from build123d import *

# Parameters (mm, degrees)
BOSS_EXTRUDE1_DEPTH = 4
BOSS_EXTRUDE2_DEPTH = 4
SKETCH3_R           = 1.25
BOSS_EXTRUDE3_DEPTH = 15
FILLET1_R           = 1
FILLET2_R           = 0.5
FILLET3_R           = 0.75


with BuildPart() as part:
    # Sketch1 → Boss-Extrude1 (new body)
    with BuildSketch(Plane.XY):
        Polygon((2.3, -4.75), (3.5, -4.75), (3.5, 4.75), (2.3, 4.75), (2.3, 2.65), (-0.2, 2.65), (-0.2, 4.75), (-3.5, 4.75), (-3.5, -4.75), (-0.2, -4.75), (-0.2, -2.65), (2.3, -2.65), align=None)
    extrude(amount=BOSS_EXTRUDE1_DEPTH)

    # Sketch2 → Boss-Extrude2 (add)
    with BuildSketch(Plane(origin=(0, 0, 0), x_dir=(-1, 0, 0), z_dir=(0, 0, -1))):
        Polygon((-7.5, 2.5), (-7.5, -2.5), (-3.5, -4.75), (-3.5, 4.75), align=None)
    extrude(amount=-BOSS_EXTRUDE2_DEPTH)

    # Sketch3 → Boss-Extrude3 (add)
    with BuildSketch(Plane.XY.offset(4)):
        with Locations((-1.5, 0)):
            Circle(SKETCH3_R)
    extrude(amount=BOSS_EXTRUDE3_DEPTH)

    # Fillet1
    fillet1_edges = [part.edges().sort_by_distance(p)[0] for p in [
        (-3.5, -4.75, 2),
        (-3.5, 4.75, 2),
        (3.5, 4.75, 2),
        (3.5, -4.75, 2),
        (7.5, -2.5, 2),
        (7.5, 2.5, 2),
    ]]
    fillet(fillet1_edges, radius=FILLET1_R)

    # Fillet2
    fillet2_edges = [part.edges().sort_by_distance(p)[0] for p in [
        (-2.75, 0, 4),
    ]]
    fillet(fillet2_edges, radius=FILLET2_R)

    # Fillet3
    fillet3_edges = [part.edges().sort_by_distance(p)[0] for p in [
        (-2.75, 0, 19),
    ]]
    fillet(fillet3_edges, radius=FILLET3_R)


solid = part.part
Geometry check sheet. Reference: the model listing, model coordinates, mm. A direction names the side the tool comes from. Round coordinates to 2 decimals unless told otherwise and drop trailing zeros. Loops run counter-clockwise (first coordinate to the right, second up) from the corner with the lowest first, then second, coordinate; pieces in that order, holes last. Notation, with made-up numbers: (18.25, 38.5) -> (77.25, 38.5) arc R22 ccw to (77.25, 47.5) -> close; hole circle Ø8 at (-32.75, 18.25). An arc over 180 degrees is marked (long way). Answer as a JSON object with one key per item and string values. Group by question number.
Item 1: Cross-section at C-C, the plane z = 14.5. Record the cut outline in (x, y).
Item 2: Cross-section at A-A, the plane z = 2.5. Record the cut outline in (x, y).
Item 3: Thickness scan on line 1 along Z through (x, y) = (4.5, 3.25); line 2 along Y through (x, z) = (-1.5, 6.25); line 3 along X through (y, z) = (-0.75, 13). Record the ranges inside material, lowest first.
Item 4: Cross-section at D-D, the plane x = 2.75. Record the cut outline in (y, z), plus the area to 3 significant figures.
Item 5: Set-up check for faces 1 (the face through (1, 2.65, 2)), 2 (the face through (3, 4.75, 2)), 3 (the face through (5.382, -3.691, 1.972)), 4 (the face through (-0.31, 0.38, 11.28)), 5 (the face through (-0.2, -4, 2)): record each of +Z, -Z, +X, -X, +Y, -Y from which the full face is reachable in a straight line by a thin tool's end or side.
Item 6: Cross-section at B-B, the plane x = 1.5. Record the cut outline in (y, z), plus the area to 3 significant figures.
Item 7: Release check for a two-part mould opening along X. For faces 6 (the face through (2, 0, 0)), 7 (the face through (2.3, -4, 2)), 8 (the face through (7.5, 0, 2)), 9 (the face through (-0.2, 4, 2)) record: pulls with the +X half, pulls with the -X half, needs draft (parallel to the pull), parting line crosses it, or undercut.
Item 8: Depth check by flat-ended pin: pin 1 Ø4 at (y, z) = (-1, 8.5) entering from +X; pin 2 Ø5 at (x, y) = (-0.5, 2) entering from +Z; pin 3 Ø2 at (x, z) = (1, 3) entering from +Y; pin 4 Ø1 at (x, y) = (-2, -1.5) entering from +Z. Enter the tip coordinate at first touch or a pass-through.
Determined:
{
 "1": {"outline": "circle Ø2.5 at (-1.5, 0)"},
 "2": {"outline": "(-3.5, -3.75) arc R1 ccw to (-2.5, -4.75) -> (-0.2, -4.75) -> (-0.2, -2.65) -> (2.3, -2.65) -> (2.3, -4.75) -> (3.24, -4.75) arc R1 ccw to (3.73, -4.62) -> (6.99, -2.79) arc R1 ccw to (7.5, -1.92) -> (7.5, 1.92) arc R1 ccw to (6.99, 2.79) -> (3.73, 4.62) arc R1 ccw to (3.24, 4.75) -> (2.3, 4.75) -> (2.3, 2.65) -> (-0.2, 2.65) -> (-0.2, 4.75) -> (-2.5, 4.75) arc R1 ccw to (-3.5, 3.75) -> close"},
 "3": {"line 1": "z = 0 to 4", "line 2": "y = -1.25 to 1.25", "line 3": "x = -2.5 to -0.5"},
 "4": {"outline": "(-4.75, 0) -> (4.75, 0) -> (4.75, 4) -> (-4.75, 4) -> close", "area": "38.0 mm²"},
 "5": {"face 1": "+Z, -Z, +Y", "face 2": "+Z, -Z, +X, -X, +Y", "face 3": "+Z, -Z, +X, -Y", "face 4": "+Z", "face 5": "+Z, -Z, -Y"},
 "6": {"outline": "(-2.65, 0) -> (2.65, 0) -> (2.65, 4) -> (-2.65, 4) -> close", "area": "21.2 mm²"},
 "7": {"face 6": "needs draft", "face 7": "undercut", "face 8": "pulls with the +X half", "face 9": "undercut"},
 "8": {"pin 1": "stops at x = -0.25", "pin 2": "stops at z = 19", "pin 3": "stops at y = 2.65", "pin 4": "stops at z = 18.72"}
}
